```python
from build123d import *

# Parameters (mm, degrees)
F0_W      = 50
F0_H      = 40
F1_DEPTH  = 40
F2_W      = 50
F2_H      = 40
F3_DEPTH  = 20
F4_W      = 10
F4_H      = 40
F5_DEPTH  = 20
F6_W      = 50
F6_H      = 10
F7_DEPTH  = 10
F8_W      = 10
F8_H      = 40
F9_DEPTH  = 20
F10_W     = 50
F10_H     = 10
F11_DEPTH = 10


with BuildPart() as f1:
    # F0 (on Front) → F1 (new body)
    with BuildSketch(Plane.XZ):
        with Locations((25, 20)):
            Rectangle(F0_W, F0_H)
    extrude(amount=F1_DEPTH)

    # F2 (on face) → F3 (cut)
    with BuildSketch(Plane.XY.offset(40)):
        with Locations((25, -20)):
            Rectangle(F2_W, F2_H)
    extrude(amount=-F3_DEPTH, mode=Mode.SUBTRACT)

    # F4 (on face) → F5 (join)
    with BuildSketch(Plane.XY.offset(20)):
        with Locations((5, -20)):
            Rectangle(F4_W, F4_H)
    extrude(amount=F5_DEPTH)

    # F6 (on face) → F7 (join)
    with BuildSketch(Plane.XY.offset(40)):
        with Locations((35, -5)):
            Rectangle(F6_W, F6_H)
    extrude(amount=-F7_DEPTH)

    # F8 (on face) → F9 (join)
    with BuildSketch(Plane.XY.offset(20)):
        with Locations((55, -20)):
            Rectangle(F8_W, F8_H)
    extrude(amount=-F9_DEPTH)

    # F10 (on face) → F11 (join)
    with BuildSketch(Plane.XZ.offset(10)):
        with Locations((35, 25)):
            Rectangle(F10_W, F10_H)
    extrude(amount=-F11_DEPTH)


solid = f1.part
```
Could you check a few things on this model? Use its own coordinates, in mm. A direction names the side the tool comes from. Round coordinates to 2 decimals unless told otherwise and drop trailing zeros. Loops run counter-clockwise (first coordinate to the right, second up) from the corner with the lowest first, then second, coordinate; pieces in that order, holes last. Notation, with made-up numbers: (-14, 13) - (15, 13) arc R25 ccw to (15, 38) - close; hole circle Ø1 at (-25.75, -32.75). An arc over 180 degrees is marked (long way). Answer in a Markdown table with one row per item. Add a question column.
(1) I'm going to push flat-ended pins straight in: pin 1 (6 mm diameter, centred on y = -29, z = 27.5, fed in from +X); pin 2 (16 mm diameter, centred on x = 32.5, z = 32.5, fed in from -Y); pin 3 (12 mm diameter, centred on x = 23.5, y = -35, fed in from +Z). Where does each tip first touch, or does it pass through?
(2) I need wall thicknesses on line 1 along Z through (x, y) = (41, -15); line 2 along Y through (x, z) = (52.5, 29.5); line 3 along X through (y, z) = (-13.5, 25.5). Which ranges of each line are inside material? Lowest first, please.
(3) If we section it at A-A (x = 29): Please give me the cut outline in (y, z), plus the area to 3 significant figures.
(4) If we section it at B-B (z = 25.5): Please give me the cut outline in (x, y).
(5) For faces 1 (the face through (30, 0, 20)), 2 (the face through (10, -25, 30)), which set-ups out of +Z, -Z, +X, -X, +Y, -Y let a thin tool reach every point of the face, with its end or its side?
Model answer:
| question | item | result |
|---|---|---|
| 1 | pin 1 | stops at x = 10 |
| 1 | pin 2 | stops at y = -10 |
| 1 | pin 3 | stops at z = 20 |
| 2 | line 1 | z = 0 to 20 |
| 2 | line 2 | y = -10 to 0 |
| 2 | line 3 | x = 0 to 10 |
| 3 | outline | (-40, 0) - (0, 0) - (0, 40) - (-10, 40) - (-10, 20) - (-40, 20) - close |
| 3 | area | 1,000 mm² |
| 4 | outline | (0, -40) - (10, -40) - (10, -10) - (60, -10) - (60, 0) - (0, 0) - close |
| 5 | face 1 | +Z, -Z, +X, -X, +Y |
| 5 | face 2 | +Z, +X, -Y |
